Work out the finished part from the listing and answer in its coordinate system (mm). Face numbers are marked on the shaded views. A direction names the side the tool comes from. Coordinates: 2 decimals unless noted, no trailing zeros. Loops run counter-clockwise (first coordinate to the right, second up) from the corner with the lowest first, then second, coordinate; pieces in that order, holes last.
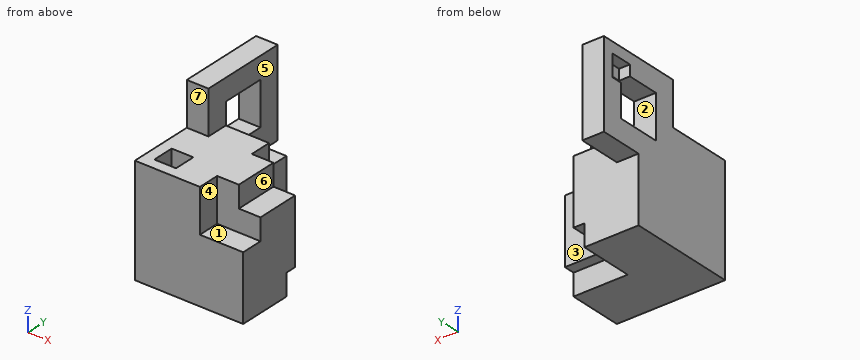
```python
from build123d import *

# Parameters (mm, degrees)
F0_W      = 25.4
F0_H      = 25.4
F1_DEPTH  = 25.4
F2_W      = 5.08
F2_H      = 5.08
F3_DEPTH  = 25.4
F4_W      = 10.16
F4_H      = 10.16
F5_DEPTH  = 5.08
F6_W      = 20.32
F6_H      = 20.32
F7_DEPTH  = 5.08
F8_W      = 10.16
F8_H      = 10.16
F9_DEPTH  = 25.4
F10_W     = 5.08
F10_H     = 5.08
F11_DEPTH = 12.7
F12_W     = 10.16
F12_H     = 10.16
F13_DEPTH = 25.4
F14_W     = 12.7
F14_H     = 12.7
F15_DEPTH = 5.08
F16_W     = 5.08
F16_H     = 5.08
F17_DEPTH = 2.54


with BuildPart() as f1:
    # F0 (on Top) → F1 (new body)
    with BuildSketch(Plane.XY):
        with Locations((12.7, 12.7)):
            Rectangle(F0_W, F0_H)
    extrude(amount=F1_DEPTH)

    # F2 (on face) → F3 (cut)
    with BuildSketch(Plane.XZ):
        with Locations((22.86, 22.86)):
            Rectangle(F2_W, F2_H)
    extrude(amount=-F3_DEPTH, mode=Mode.SUBTRACT)

    # F4 (on face) → F5 (cut)
    with BuildSketch(Plane.XZ):
        with Locations((20.32, 20.32)):
            Rectangle(F4_W, F4_H)
    extrude(amount=-F5_DEPTH, mode=Mode.SUBTRACT)

    # F6 (on face) → F7 (join)
    with BuildSketch(Plane(origin=(0, 0, 0), x_dir=(0, -1, 0), z_dir=(-1, 0, 0))):
        with Locations((-25.4, 25.4)):
            Rectangle(F6_W, F6_H)
    extrude(amount=-F7_DEPTH)

    # F8 (on face) → F9 (cut)
    with BuildSketch(Plane(origin=(0, 0, 0), x_dir=(0, -1, 0), z_dir=(-1, 0, 0))):
        with Locations((-25.4, 25.4)):
            Rectangle(F8_W, F8_H)
    extrude(amount=-F9_DEPTH, mode=Mode.SUBTRACT)

    # F10 (on face) → F11 (cut)
    with BuildSketch(Plane.XY.offset(25.4)):
        with Locations((5.08, 5.08)):
            Rectangle(F10_W, F10_H)
    extrude(amount=-F11_DEPTH, mode=Mode.SUBTRACT)

    # F12 (on face) → F13 (cut)
    with BuildSketch(Plane.XY.offset(25.4)):
        with Locations((20.32, 20.32)):
            Rectangle(F12_W, F12_H)
    extrude(amount=-F13_DEPTH, mode=Mode.SUBTRACT)

    # F14 (on face) → F15 (cut)
    with BuildSketch(Plane(origin=(0, 0, 0), x_dir=(1, 0, 0), z_dir=(0, 0, -1))):
        with Locations((19.05, -19.05)):
            Rectangle(F14_W, F14_H)
    extrude(amount=-F15_DEPTH, mode=Mode.SUBTRACT)

    # F16 (on face) → F17 (cut)
    with BuildSketch(Plane(origin=(0, 0, 0), x_dir=(0, -1, 0), z_dir=(-1, 0, 0))):
        with Locations((-30.48, 30.48)):
            Rectangle(F16_W, F16_H)
    extrude(amount=-F17_DEPTH, mode=Mode.SUBTRACT)


solid = f1.part
```
1. Determine the mould class of the marked faces 1, 2 and 3 for opening direction Y: released by +Y, released by -Y, zero draft, split by the parting line, or undercut.
2. A cutting plane is placed at B-B, the plane y = 21.5. Give the vertices of the cut face in (x, z).
3. A cutting plane is placed at D-D, the plane x = 21.5. Give the vertices of the cut face in (y, z), then the cut area to 3 significant figures.
4. Each of these flat-tipped pins is pushed along its axis until it touches: P1, Ø5, axis at x = 8.5, z = 27, coming from the +Y side; P2, Ø5.5, axis at x = 16.5, z = 3.5, coming from the +Y side; P3, Ø5.5, axis at x = 22.5, y = 2, coming from the +Z side. Where does it stop, or does it pass through?
5. For the marked faces 4, 5, 6 and 7, determine the directions among +Z, -Z, +X, -X, +Y, -Y from which every point of the face is accessible in a straight line to the end or side of a thin tool.
6. A cutting plane is placed at C-C, the plane x = 3. Give the vertices of the cut face in (y, z), then the cut area to 3 significant figures.
7. A cutting plane is placed at A-A, the plane z = 29. Give the vertices of the cut face in (x, y).
8. Straight lines are drawn through the part: probe 1 along X at (y, z) = (3, 18.5); probe 2 along Z at (x, y) = (20.25, 7); probe 3 along X at (y, z) = (31.5, 22). For each, find the intervals that lie inside material, in ascending order.
Answers below:
1. face 1: zero draft
1. face 2: undercut
1. face 3: released by +Y
2. outline: (0, 0) - (12.7, 0) - (12.7, 5.08) - (15.24, 5.08) - (15.24, 20.32) - (0, 20.32) - close; (0, 30.48) - (5.08, 30.48) - (5.08, 35.56) - (0, 35.56) - close
3. outline: (0, 0) - (12.7, 0) - (12.7, 5.08) - (15.24, 5.08) - (15.24, 20.32) - (5.08, 20.32) - (5.08, 15.24) - (0, 15.24) - close
3. area: 271 mm2
4. P1: stops at y = 20.32
4. P2: stops at y = 25.4
4. P3: stops at z = 15.24
5. face 4: +Z, +X, -Y
5. face 5: +Z, +X, +Y
5. face 6: +Z, +X, +Y, -Y
5. face 7: +Z, +X, -X, -Y
6. outline: (0, 0) - (25.4, 0) - (25.4, 15.24) - (35.56, 15.24) - (35.56, 35.56) - (15.24, 35.56) - (15.24, 25.4) - (7.62, 25.4) - (7.62, 12.7) - (2.54, 12.7) - (2.54, 25.4) - (0, 25.4) - close; hole (20.32, 20.32) - (30.48, 20.32) - (30.48, 30.48) - (20.32, 30.48) - close
6. area: 787 mm2
7. outline: (0, 15.24) - (5.08, 15.24) - (5.08, 20.32) - (0, 20.32) - close; (0, 33.02) - (2.54, 33.02) - (2.54, 30.48) - (5.08, 30.48) - (5.08, 35.56) - (0, 35.56) - close
8. probe 1: x = 0 to 2.54, 7.62 to 15.24
8. probe 2: z = 0 to 25.4
8. probe 3: x = 0 to 5.08
